from build123d import *

# Parameters (mm, degrees)
F0_R     = 3.175
F1_DEPTH = 3.048


with BuildPart() as f1:
    # F0 (on Front) → F1 (new body)
    with BuildSketch(Plane.XZ):
        with BuildLine():
            ThreePointArc((44.811011276, -7.9292860403), (50.1888776452, -5.4835380571), (52.3875, 0))
            ThreePointArc((52.3875, 0), (47.9572367593, 7.1206177094), (39.611891417, 6.2925838563))
            ThreePointArc((39.611891417, 6.2925838563), (36.9950354855, -2.7253275651), (44.811011276, -7.9292860403))
        make_face()
        with Locations((44.2953519523, -0.143149824)):
            Circle(F0_R, mode=Mode.SUBTRACT)
        with BuildLine():
            ThreePointArc((44.811011276, -7.9292860403), (36.9950354855, -2.7253275651), (39.611891417, 6.2925838563))
            Line((39.611891417, 6.2925838563), (18.3958708033, 7.7857948995))
            ThreePointArc((18.3958708033, 7.7857948995), (12.8944465004, 10.5698187456), (11.0376963734, 16.4493541951))
            Line((11.0376963734, 16.4493541951), (14.947713815, 58.6785307391))
            ThreePointArc((14.947713815, 58.6785307391), (-0.1463299689, 47.6247825372), (-15.2836352123, 58.6192128102))
            Line((-15.2836352123, 58.6192128102), (-9.969479858, 0))
            ThreePointArc((-9.969479858, 0), (0, 9.969479858), (9.969479858, 0))
            ThreePointArc((9.969479858, 0), (7.3628146901, -6.7215689001), (0.905920049, -9.9282343598))
            Line((0.905920049, -9.9282343598), (44.811011276, -7.9292860403))
        make_face()
        with BuildLine():
            ThreePointArc((0, -9.969479858), (0.4534292465, -9.9591631454), (0.905920049, -9.9282343598))
            Line((0.905920049, -9.9282343598), (0, -9.969479858))
        make_face()
        with BuildLine():
            Line((0, -9.969479858), (0.905920049, -9.9282343598))
            ThreePointArc((0.905920049, -9.9282343598), (7.3628146901, -6.7215689001), (9.969479858, 0))
            ThreePointArc((9.969479858, 0), (0, 9.969479858), (-9.969479858, 0))
            ThreePointArc((-9.969479858, 0), (-7.0494868125, -7.0494868125), (0, -9.969479858))
        make_face()
        Circle(F0_R, mode=Mode.SUBTRACT)
        with BuildLine():
            Line((15.5757910153, 65.4619232349), (14.947713815, 58.6785307391))
            ThreePointArc((14.947713815, 58.6785307391), (15.5089493964, 61.060162597), (15.697521229, 63.4997519781))
            ThreePointArc((15.697521229, 63.4997519781), (15.6670594498, 64.4827237842), (15.5757910153, 65.4619232349))
        make_face()
        with BuildLine():
            ThreePointArc((-15.2836352123, 58.6192128102), (-0.1463299689, 47.6247825372), (14.947713815, 58.6785307391))
            Line((14.947713815, 58.6785307391), (15.5757910153, 65.4619232349))
            ThreePointArc((15.5757910153, 65.4619232349), (-0.1158692301, 79.374632427), (-15.9150440924, 65.5841374399))
            Line((-15.9150440924, 65.5841374399), (-15.2836352123, 58.6192128102))
        make_face()
        with Locations((-0.3013272653, 63.1359219551)):
            Circle(F0_R, mode=Mode.SUBTRACT)
        with BuildLine():
            ThreePointArc((-15.9150440924, 65.5841374399), (-15.9876443874, 62.0664731565), (-15.2836352123, 58.6192128102))
            Line((-15.2836352123, 58.6192128102), (-15.9150440924, 65.5841374399))
        make_face()
        with BuildLine():
            ThreePointArc((-15.9150440924, 65.5841374399), (-0.1158692301, 79.374632427), (15.5757910153, 65.4619232349))
            Line((15.5757910153, 65.4619232349), (9.5149043603, 114.1216833297))
            ThreePointArc((9.5149043603, 114.1216833297), (0.1285774786, 104.7759850451), (-9.522687446, 113.8478257686))
            Line((-9.522687446, 113.8478257686), (-15.9150440924, 65.5841374399))
        make_face()
        with Locations((-1.5948739996, 100.0249519781)):
            Circle(F0_R, mode=Mode.SUBTRACT)
        with BuildLine():
            ThreePointArc((-9.522687446, 113.8478257686), (0.1285774786, 104.7759850451), (9.5149043603, 114.1216833297))
            ThreePointArc((9.5149043603, 114.1216833297), (9.5161563004, 114.210837603), (9.516573626, 114.2999996894))
            ThreePointArc((9.516573626, 114.2999996894), (-0.2345770866, 123.8223145789), (-9.522687446, 113.8478257686))
        make_face()
        with Locations((-0.3013272653, 114.663168788)):
            Circle(F0_R, mode=Mode.SUBTRACT)
    extrude(amount=F1_DEPTH)


solid = f1.part
Verification items for the finished model (mm, model axes). A direction names the side the tool comes from. Give positions to 0.01 mm unless a question says otherwise; leave off trailing zeros. Write each loop counter-clockwise with the first axis right and the second up, starting at its lowest first coordinate (ties: lowest second). Pieces come first, ordered by that corner, then holes.
(1) Cross-section at A-A (y = -1.45). State how many separate pieces and enclosed holes the cut face has, plus the area to 3 significant figures.
(2) Cross-section at B-B (x = 42.5). Enter the section's corners in (y, z).
(3) Mould release check, pull along X, two halves, no side actions. Record for faces 1 (the face through (29.15, -1.5, 7.03)), 2 (the face through (22.551, -1.503, -8.943)), 3 (the face through (2, 0, 43)), 4 (the face through (-15.992, -1.503, 62.116)): +X half, -X half, draft (parallel to the pull), parting line (faces both ways), or undercut.
(4) Cross-section at D-D (z = 85). Enter the section's corners in (x, y), plus the area to 3 significant figures.
(5) Cross-section at C-C (x = -1.5). Enter the section's corners in (y, z), plus the area to 3 significant figures.
(6) Access from +Z, -Z, +X, -X, +Y, -Y to the whole of each face (thin tool, end or side, straight path). Record for faces 5 (the face through (12.965, -1.503, 37.268)), 6 (the face through (-12.674, -1.503, 90.054)).
(7) Gauge pin test, flat ends, axial feed: pin 1 (1 mm diameter, centred on y = -1, z = 18.5, fed in from -X); pin 2 (1.5 mm diameter, centred on y = -2, z = 107.5, fed in from +X). Record the tip position at first contact, or that the pin passes through.
(8) Material ranges on line 1 (Z direction, x = -4, y = -0.25); line 2 (X direction, y = -0.55, z = 117.5); line 3 (Z direction, x = 29, y = -2.35), recorded low to high.
Worked out:
1. separate pieces: 1
1. enclosed holes: 5
1. area: 3,730 mm2
2. outline: (-3.05, -8.03) - (0, -8.03) - (0, -2.76) - (-3.05, -2.76) - close; (-3.05, 2.48) - (0, 2.48) - (0, 7.69) - (-3.05, 7.69) - close
3. face 1: undercut
3. face 2: +X half
3. face 3: draft
3. face 4: -X half
4. outline: (-13.34, -3.05) - (13.14, -3.05) - (13.14, 0) - (-13.34, 0) - close
4. area: 80.7 mm2
5. outline: (-3.05, -9.86) - (0, -9.86) - (0, -2.8) - (-3.05, -2.8) - close; (-3.05, 2.8) - (0, 2.8) - (0, 60.2) - (-3.05, 60.2) - close; (-3.05, 66.08) - (0, 66.08) - (0, 96.85) - (-3.05, 96.85) - close; (-3.05, 103.2) - (0, 103.2) - (0, 111.72) - (-3.05, 111.72) - close; (-3.05, 117.6) - (0, 117.6) - (0, 123.71) - (-3.05, 123.71) - close
5. area: 335 mm2
6. face 5: +X, +Y, -Y
6. face 6: +Z, -X, +Y, -Y
7. pin 1: stops at x = -11.69
7. pin 2: stops at x = 10.43
8. line 1: z = -9.13 to 97.95, 102.1 to 122.95
8. line 2: x = -8.98 to -1.73, 1.12 to 8.96
8. line 3: z = -8.65 to 7.04
